```python
from build123d import *

# Parameters (mm, degrees)
SKETCH_1_R      = 2
EXTRUDE_1_DEPTH = 5
CHAMFER_1_SIZE  = 0.5


with BuildPart() as part:
    # 草图1 → 凸台-拉伸1 (new body)
    with BuildSketch(Plane(origin=(0, 0, 0), x_dir=(1, 0, 0), z_dir=(0, 1, 0))):
        Polygon((-3.983716857, 0), (-1.991858429, -3.45), (1.991858429, -3.45), (3.983716857, 0), (1.991858429, 3.45), (-1.991858429, 3.45), align=None)
        with Locations(Location((0, 0, 0), (0, 0, 270))):
            Circle(SKETCH_1_R, mode=Mode.SUBTRACT)
    extrude(amount=EXTRUDE_1_DEPTH)

    # 倒角1
    chamfer_1_edges = [part.edges().sort_by_distance(p)[0] for p in [
        (0, 5, 3.45),
        (2.987787643, 5, 1.725),
        (2.987787643, 5, -1.725),
        (0, 5, -3.45),
        (-2.987787643, 5, -1.725),
        (0, 0, -3.45),
        (2.987787643, 0, -1.725),
        (2.987787643, 0, 1.725),
        (0, 0, 3.45),
        (-2.987787643, 0, 1.725),
        (-2.987787643, 0, -1.725),
        (-2.987787643, 5, 1.725),
    ]]
    chamfer(chamfer_1_edges, length=CHAMFER_1_SIZE)


solid = part.part
```
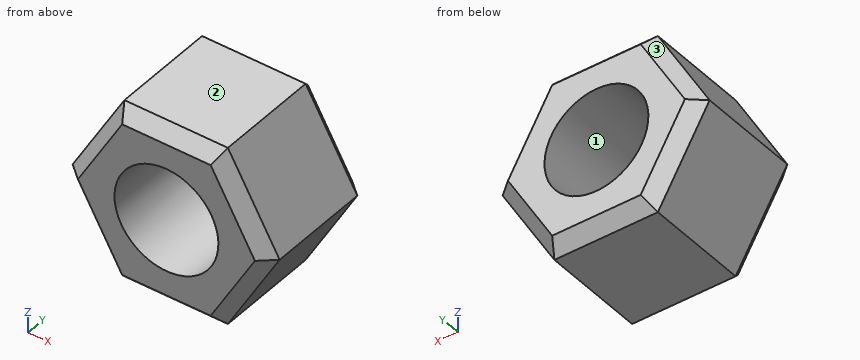
Work out the finished part from the listing and answer in its coordinate system (mm). Face numbers are marked on the shaded views. Round coordinates to 2 decimals unless told otherwise and drop trailing zeros. Loops run counter-clockwise (first coordinate to the right, second up) from the corner with the lowest first, then second, coordinate; pieces in that order, holes last. Notation, with made-up numbers: M 85.5,48 L 92.5,48 A23 cw 92.5,63 Z; hole C -21.5,31 d7. An arc over 180 degrees is marked long. One line per question, with ' | ' between items.
Q1. This flat-tipped pin is pushed along its axis until it touches: pin 1 Ø1.5 at (y, z) = (4, -2) entering from -X. Where does it stop, or does it pass through?
Conclusion:
pin 1: stops at x = -3.26
Q2. Find section D-D, the plane x = 3.25. Give the vertices of the cut face in (y, z).
Conclusion:
outline: M 0,-0.27 L 0.5,-1.27 L 4.5,-1.27 L 5,-0.27 L 5,0.27 L 4.5,1.27 L 0.5,1.27 L 0,0.27 Z
Q3. Find section A-A, the plane x = 0. Give the vertices of the cut face in (y, z).
Conclusion:
outline: M 0,-2.95 L 0.5,-3.45 L 4.5,-3.45 L 5,-2.95 L 5,-2 L 0,-2 Z; M 0,2 L 5,2 L 5,2.95 L 4.5,3.45 L 0.5,3.45 L 0,2.95 Z
Q4. Find section C-C, the plane y = 3.05. Give the vertices of the cut face in (x, z), then the cut area to 3 significant figures.
Conclusion:
outline: M -3.98,0 L -1.99,-3.45 L 1.99,-3.45 L 3.98,0 L 1.99,3.45 L -1.99,3.45 Z; hole C 0,0 d4 | area: 28.7 mm2
Q5. Find section B-B, the plane z = 1.25. Give the vertices of the cut face in (x, y), then the cut area to 3 significant figures.
Conclusion:
outline: M -3.26,0.5 L -2.68,0 L -1.56,0 L -1.56,5 L -2.68,5 L -3.26,4.5 Z; M 1.56,0 L 2.68,0 L 3.26,0.5 L 3.26,4.5 L 2.68,5 L 1.56,5 Z | area: 16.4 mm2
Q6. The mould has two halves that part along X. Classify the marked faces 1, 2 and 3: +X half, -X half, draft (parallel to the pull), parting line (faces both ways), or undercut.
Conclusion:
face 1: undercut | face 2: draft | face 3: -X half
Q7. Consider line 1 along Z through (x, y) = (-0.5, 0.3); line 2 along Z through (x, y) = (3, 2.45); line 3 along Z through (x, y) = (-1.5, 2.75). Determine where each line is inside the solid, lowest interval first. Write a range as from..to.
Conclusion:
line 1: z = -3.25..-1.94, 1.94..3.25 | line 2: z = -1.7..1.7 | line 3: z = -3.45..-1.32, 1.32..3.45
